Could you check a few things on this model? Use its own coordinates, in mm. Face numbers are marked on the shaded views. A direction names the side the tool comes from. Coordinates: 2 decimals unless noted, no trailing zeros. Order: outer loops, then holes, each group sorted by start corner. A loop starts at its lowest first (then second) coordinate and runs counter-clockwise, first axis right, second up. Notation, with made-up numbers: (-17, 88.5) - (24, 88.5) arc R16 ccw to (24, 93.5) - close; hole circle Ø3 at (-3, 33). An arc over 180 degrees is marked (long way). Answer as CSV lines item,"result". Start each with the question number.
1. Thinking about a two-plate mould opening in Z: for the marked faces 1, 2 and 3, which applies, released by +Z, released by -Z, zero draft, split by the parting line, or undercut?
2. I need wall thicknesses on probe 1 along Z at (x, y) = (18, 24); probe 2 along Y at (x, z) = (18, 23); probe 3 along Y at (x, z) = (16, 32.5). Which ranges of each line are inside material? Lowest first, please.
3. I want a section at A-A, the plane z = 4. List the corners of the cut face in (x, y) for me, and give its area (3 significant figures).
4. For the marked faces 4 and 5, which set-ups out of +Z, -Z, +X, -X, +Y, -Y let a thin tool reach every point of the face, with its end or its side?
5. I want a section at C-C, the plane x = 23.5. List the corners of the cut face in (y, z) for me.
6. For pin 1 (1.5 mm diameter, centred on y = 32.5, z = 25, fed in from -X); pin 2 (6 mm diameter, centred on x = 9, z = 24, fed in from +Y); pin 3 (6 mm diameter, centred on x = 23, z = 16, fed in from +Y), each with a flat end and sliding along its axis, tell me the tip position at first contact or that it passes through.
7. I want a section at B-B, the plane y = 22.5. List the corners of the cut face in (x, z) for me.
8. I want a section at D-D, the plane z = 20. List the corners of the cut face in (x, y) for me, and give its area (3 significant figures).
from build123d import *

# Parameters (mm, degrees)
SKETCH1_W           = 40
SKETCH1_H           = 40
BOSS_EXTRUDE1_DEPTH = 40
CUT_EXTRUDE1_DEPTH  = 40
CUT_EXTRUDE2_DEPTH  = 20
CUT_EXTRUDE3_DEPTH  = 30
BOSS_EXTRUDE2_DEPTH = 10
BOSS_EXTRUDE3_DEPTH = 20


with BuildPart() as part:
    # Sketch1 → Boss-Extrude1 (new body)
    with BuildSketch(Plane.XY):
        with Locations((20, 20)):
            Rectangle(SKETCH1_W, SKETCH1_H)
    extrude(amount=BOSS_EXTRUDE1_DEPTH)

    # Sketch2 → Cut-Extrude1 (cut)
    with BuildSketch(Plane.XY.offset(40)):
        with BuildLine():
            Line((0, 40), (0, 20))
            ThreePointArc((0, 20), (5.857864376, 34.142135624), (20, 40))
            Line((20, 40), (0, 40))
        make_face()
        with BuildLine():
            Line((40, 40), (20, 40))
            ThreePointArc((20, 40), (34.142135624, 34.142135624), (40, 20))
            Line((40, 20), (40, 40))
        make_face()
    extrude(amount=-CUT_EXTRUDE1_DEPTH, mode=Mode.SUBTRACT)

    # Sketch3 → Cut-Extrude2 (cut)
    with BuildSketch(Plane.XY.offset(10)):
        with BuildLine():
            Line((0, 20), (20, 20))
            Line((20, 20), (20, 40))
            ThreePointArc((20, 40), (5.857864376, 34.142135624), (0, 20))
        make_face()
    extrude(amount=CUT_EXTRUDE2_DEPTH, mode=Mode.SUBTRACT)

    # Sketch4 → Cut-Extrude3 (cut)
    with BuildSketch(Plane.XY.offset(40)):
        with BuildLine():
            Line((20, 20), (20, 40))
            ThreePointArc((20, 40), (27.653668647, 38.47759065), (34.142135624, 34.142135624))
            Line((34.142135624, 34.142135624), (20, 20))
        make_face()
    extrude(amount=-CUT_EXTRUDE3_DEPTH, mode=Mode.SUBTRACT)

    # Sketch5 → Boss-Extrude2 (add)
    with BuildSketch(Plane.XY.offset(40)):
        with BuildLine():
            Line((20, 40), (20, 20))
            Line((20, 20), (34.142135624, 34.142135624))
            ThreePointArc((34.142135624, 34.142135624), (27.653668647, 38.47759065), (20, 40))
        make_face()
    extrude(amount=-BOSS_EXTRUDE2_DEPTH)

    # Sketch6 → Boss-Extrude3 (add)
    with BuildSketch(Plane.XY.offset(10)):
        with BuildLine():
            Line((20, 20), (34.142135624, 34.142135624))
            ThreePointArc((34.142135624, 34.142135624), (32.17522858, 35.867066806), (30, 37.320508076))
            Line((30, 37.320508076), (20, 20))
        make_face()
    extrude(amount=BOSS_EXTRUDE3_DEPTH)


solid = part.part
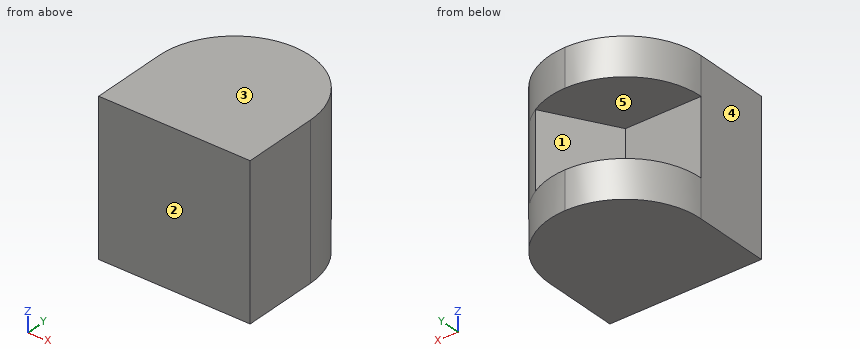
Solved:
1,face 1,"undercut"
1,face 2,"zero draft"
1,face 3,"released by +Z"
2,probe 1,"z = 0 to 10, 30 to 40"
2,probe 2,"y = 0 to 20"
2,probe 3,"y = 0 to 39.6"
3,outline,"(0, 0) - (40, 0) - (40, 20) arc R20 ccw to (0, 20) - close"
3,area,"1,430 mm2"
4,face 4,"+Z, -Z, -X, +Y, -Y"
4,face 5,"-X, +Y"
5,outline,"(0, 0) - (39.69, 0) - (39.69, 10) - (26.06, 10) - (26.06, 30) - (39.69, 30) - (39.69, 40) - (0, 40) - close"
6,pin 1,"stops at x = 26.78"
6,pin 2,"stops at y = 20"
6,pin 3,"stops at y = 30.39"
7,outline,"(0.16, 0) - (39.84, 0) - (39.84, 40) - (0.16, 40) - (0.16, 30) - (21.44, 30) - (21.44, 10) - (0.16, 10) - close"
8,outline,"(0, 0) - (40, 0) - (40, 20) arc R20 ccw to (30, 37.32) - (20, 20) - (0, 20) - close"
8,area,"1,010 mm2"
